For this review, take the finished solid that the model builds, in its own axes (mm). A direction names the side the tool comes from. Round coordinates to 2 decimals unless told otherwise and drop trailing zeros. Order: outer loops, then holes, each group sorted by start corner. A loop starts at its lowest first (then second) coordinate and runs counter-clockwise, first axis right, second up. Notation, with made-up numbers: (38, 34) -> (90, 34) arc R19 ccw to (90, 69) -> close; hole circle Ø5 at (52, -5). An arc over 180 degrees is marked (long way). Use a Markdown table: item, result. Add a question column.
1) Clearance check with flat-ended pins moving along their axes: P1, Ø2, axis at y = -2, z = -8.5, coming from the -X side; P2, Ø3, axis at x = 1.5, y = -1, coming from the -Z side; P3, Ø1, axis at x = 0, z = -9.5, coming from the +Y side. State where each tip first meets the part, or that it passes through.
2) Machinability: for faces 1 (the face through (-0.63, -1.08, 1.36)), 2 (the face through (1.2, -1.2, 0)), 3 (the face through (-0.596, -2.685, 0.838)), which of the approach directions +Z, -Z, +X, -X, +Y, -Y give a long, thin tool a straight path to every point of the face, cutting with its end or side? Answer none if there is none.
3) Consider section B-B (z = -9). State the section outline as (x, y) points.
4) Draft analysis for pull direction Y (two halves, no side actions). For faces 4 (the face through (1.25, 0, 1)), 5 (the face through (1.1, -1.1, 2)), 6 (the face through (-1.5, -0.07, -5.92)), state which applies: pulls with the +Y half, pulls with the -Y half, needs draft (parallel to the pull), parting line crosses it, or undercut.
5) Wall thickness on line 1 along X through (y, z) = (-0.05, 1.5); line 2 along Z through (x, y) = (0.6, -2.3); line 3 along Z through (x, y) = (-0.95, -0.85): over which ranges is each line inside the solid? List them lowest first. Write a range as [from, to].
6) Consider section A-A (y = 0). State the section outline as (x, z) points.
```python
from build123d import *

# Parameters (mm, degrees)
F0_R     = 2.75
F1_DEPTH = 2
F3_DEPTH = 1.3
F4_R     = 1.5
F5_DEPTH = 12
F6_R     = 0.3


with BuildPart() as f1:
    # F0 (on Top) → F1 (new body)
    with BuildSketch(Plane.XY):
        Circle(F0_R)
    extrude(amount=F1_DEPTH)

    # F2 (on face) → F3 (cut)
    with BuildSketch(Plane.XY.offset(2)):
        Polygon((1.25, -0.721688), (1.25, 0.721688), (0, 1.443376), (-1.25, 0.721688), (-1.25, -0.721688), (0, -1.443376), align=None)
    extrude(amount=-F3_DEPTH, mode=Mode.SUBTRACT)

    # F4 (on face) → F5 (join)
    with BuildSketch(Plane(origin=(0, 0, 0), x_dir=(1, 0, 0), z_dir=(0, 0, -1))):
        Circle(F4_R)
    extrude(amount=F5_DEPTH)

    # F6
    f6_edges = [f1.edges().sort_by_distance(p)[0] for p in [
        (-2.75, 0, 2),
    ]]
    fillet(f6_edges, radius=F6_R)


solid = f1.part
```
Results list:
| question | item | result |
|---|---|---|
| 1 | P1 | x = -1.12 |
| 1 | P2 | z = -12 |
| 1 | P3 | y = 1.5 |
| 2 | face 1 | +Z |
| 2 | face 2 | -Z |
| 2 | face 3 | +Z, -Z |
| 3 | outline | circle Ø3 at (0, 0) |
| 4 | face 4 | undercut |
| 4 | face 5 | needs draft |
| 4 | face 6 | parting line crosses it |
| 5 | line 1 | [-2.75, -1.25], [1.25, 2.75] |
| 5 | line 2 | [0, 2] |
| 5 | line 3 | [-12, 0.7] |
| 6 | outline | (-2.75, 0) -> (-1.5, 0) -> (-1.5, -12) -> (1.5, -12) -> (1.5, 0) -> (2.75, 0) -> (2.75, 1.7) arc R0.3 ccw to (2.45, 2) -> (1.25, 2) -> (1.25, 0.7) -> (-1.25, 0.7) -> (-1.25, 2) -> (-2.45, 2) arc R0.3 ccw to (-2.75, 1.7) -> close |
